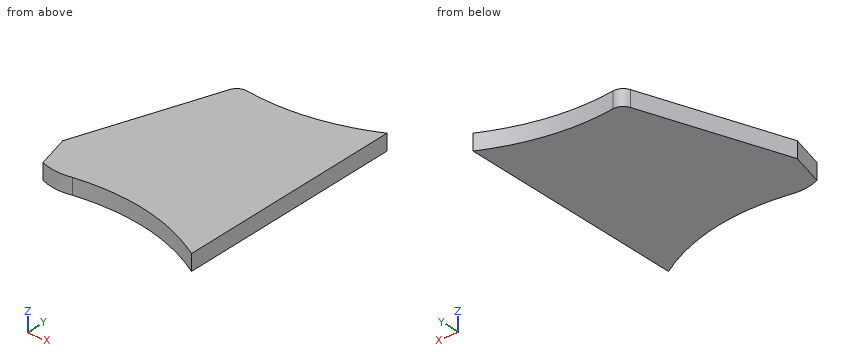
from build123d import *

# Parameters (mm, degrees)
EXTRUDE_1_DEPTH      = 3
EXTRUDE_2_DEPTH      = 3
CUT_EXTRUDE_1_DEPTH  = 10
CUT_EXTRUDE_2_DEPTH  = 10
FILLET_1_R           = 2
CUT_EXTRUDE_3_DEPTH  = 10
CUT_EXTRUDE_4_DEPTH  = 10
CUT_EXTRUDE_5_DEPTH  = 10
CUT_EXTRUDE_6_DEPTH  = 10
CUT_EXTRUDE_7_DEPTH  = 10
EXTRUDE_3_DEPTH      = 3
EXTRUDE_4_DEPTH      = 3
EXTRUDE_5_DEPTH      = 3
CUT_EXTRUDE_8_DEPTH  = 10
CUT_EXTRUDE_9_DEPTH  = 10
CUT_EXTRUDE_10_DEPTH = 10
EXTRUDE_7_DEPTH      = 3
CUT_EXTRUDE_11_DEPTH = 10
CUT_EXTRUDE_12_DEPTH = 10
CUT_EXTRUDE_13_DEPTH = 10
FILLET_2_R           = 2


with BuildPart() as part:
    # 草图1 → 凸台-拉伸1 (new body)
    with BuildSketch(Plane.XY):
        Polygon((18.419709666, -31.180034248), (-18.99770992, -2.648675004), (-11.516544217, 31.616418832), (-4.12729008, 31.616418832), (18.99770992, 31.616418832), (18.99770992, -31.616418832), align=None)
    extrude(amount=EXTRUDE_1_DEPTH)

    # 草图2 → 凸台-拉伸2 (add)
    with BuildSketch(Plane.XY.offset(3)):
        Polygon((18.99770992, 31.616418832), (18.99770992, 39.616418832), (-11.516544217, 31.616418832), align=None)
    extrude(amount=-EXTRUDE_2_DEPTH)

    # 草图3 → 切除-拉伸1 (cut)
    with BuildSketch(Plane.XY.offset(3)):
        with BuildLine():
            Line((-18.99770992, -2.648675004), (18.419709666, -31.180034248))
            Line((18.419709666, -31.180034248), (18.99770992, -31.616418832))
            add(Edge.make_bspline(
                [(-18.99770992, -2.648675004), (-4.909401081, -6.664762391), (12.96021978, -16.653979791), (18.99770992, -31.616418832)],
                knots=[0, 0, 0, 0, 0.839418351, 0.839418351, 0.839418351, 0.839418351], degree=3))
        make_face()
    extrude(amount=-CUT_EXTRUDE_1_DEPTH, mode=Mode.SUBTRACT)

    # 草图4 → 切除-拉伸2 (cut)
    with BuildSketch(Plane.XY.offset(3)):
        with BuildLine():
            Line((18.99770992, 39.616418832), (-11.516544217, 31.616418832))
            add(Edge.make_bspline(
                [(-11.516544217, 31.616418832), (5.451208804, 29.787696143), (18.99770992, 39.616418832)],
                knots=[0, 0, 0, 1, 1, 1], degree=2))
        make_face()
    extrude(amount=-CUT_EXTRUDE_2_DEPTH, mode=Mode.SUBTRACT)

    # 圆角1
    fillet_1_edges = [part.edges().sort_by_distance(p)[0] for p in [
        (-11.516544217, 31.616418832, 1.5),
        (-18.99770992, -2.648675004, 1.5),
    ]]
    fillet(fillet_1_edges, radius=FILLET_1_R)

    # 草图5 → 切除-拉伸3 (cut)
    with BuildSketch(Plane.XY.offset(3)):
        with BuildLine():
            Line((-15.247678714, 14.527147092), (-18.602325656, -0.837743464))
            ThreePointArc((-18.602325656, -0.837743464), (-18.37793511, -2.26862535), (-17.246477615, -3.172825565))
            add(Edge.make_bspline(
                [(-5.349580984, -8.035622202), (-9.34088255, -6.003793842), (-13.405831379, -4.376501244), (-17.246477615, -3.172825565)],
                knots=[0.580679004, 0.580679004, 0.580679004, 0.580679004, 0.804994854, 0.804994854, 0.804994854, 0.804994854], degree=3))
            Line((-5.349580984, -8.035622202), (-15.247678714, 14.527147092))
        make_face()
    extrude(amount=-CUT_EXTRUDE_3_DEPTH, mode=Mode.SUBTRACT)

    # 草图6 → 切除-拉伸4 (cut)
    with BuildSketch(Plane.XY.offset(3)):
        with BuildLine():
            Line((18.99770992, -31.616418832), (18.99770992, -24.041974817))
            add(Edge.make_bspline(
                [(-5.349580984, -8.035622202), (10.712822768, -10.603879461), (18.99770992, -24.041974817)],
                knots=[0, 0, 0, 1, 1, 1], degree=2))
            add(Edge.make_bspline(
                [(18.99770992, -31.616418832), (14.821194408, -21.265949132), (4.982569087, -13.295348934), (-5.349580984, -8.035622202)],
                knots=[0, 0, 0, 0, 0.580679004, 0.580679004, 0.580679004, 0.580679004], degree=3))
        make_face()
    extrude(amount=-CUT_EXTRUDE_4_DEPTH, mode=Mode.SUBTRACT)

    # 草图7 → 切除-拉伸5 (cut)
    with BuildSketch(Plane.XY.offset(3)):
        with BuildLine():
            Line((-7.501131826, -3.13114999), (-5.349580984, -8.035622202))
            add(Edge.make_bspline(
                [(18.99770992, -24.041974817), (10.712822768, -10.603879461), (-5.349580984, -8.035622202)],
                knots=[0, 0, 0, 1, 1, 1], degree=2))
            Line((18.99770992, -24.041974817), (18.99770992, -15.72868914))
            add(Edge.make_bspline(
                [(-7.501131826, -3.13114999), (8.534248318, -3.706395951), (18.99770992, -15.72868914)],
                knots=[0, 0, 0, 1, 1, 1], degree=2))
        make_face()
    extrude(amount=-CUT_EXTRUDE_5_DEPTH, mode=Mode.SUBTRACT)

    # 草图9 → 切除-拉伸6 (cut)
    with BuildSketch(Plane.XY.offset(3)):
        with BuildLine():
            Line((-15.247678714, 14.527147092), (-5.393109321, 31.338029381))
            add(Edge.make_bspline(
                [(-9.792557358, 31.460050353), (-7.562671253, 31.296266706), (-5.393109321, 31.338029381)],
                knots=[0, 0, 0, 1, 1, 1], degree=2))
            ThreePointArc((-9.792557358, 31.460050353), (-11.135472525, 31.068108787), (-11.893031771, 29.892037648))
            Line((-11.893031771, 29.892037648), (-15.247678714, 14.527147092))
        make_face()
    extrude(amount=-CUT_EXTRUDE_6_DEPTH, mode=Mode.SUBTRACT)

    # 草图10 → 切除-拉伸7 (cut)
    with BuildSketch(Plane.XY.offset(3)):
        Polygon((-15.247678714, 14.527147092), (-5.393109321, 31.338029381), (-13.423981873, 10.370019914), align=None)
    extrude(amount=-CUT_EXTRUDE_7_DEPTH, mode=Mode.SUBTRACT)

    # 草图11 → 凸台-拉伸3 (add)
    with BuildSketch(Plane.XY.offset(3)):
        Polygon((-13.423981873, 3.619434962), (-7.501131826, -3.13114999), (-13.423981873, 10.370019914), align=None)
        Polygon((-13.423981873, 16.619434962), (-13.423981873, 10.370019914), (-5.393109321, 31.338029381), align=None)
    extrude(amount=-EXTRUDE_3_DEPTH)

    # 草图12 → 凸台-拉伸4 (add)
    with BuildSketch(Plane.XY.offset(3)):
        with BuildLine():
            Line((18.99770992, -15.72868914), (18.99770992, -16.37868914))
            add(Edge.make_bspline(
                [(-7.501131826, -3.13114999), (8.231572952, -4.86202672), (18.99770992, -16.37868914)],
                knots=[0, 0, 0, 1, 1, 1], degree=2))
            add(Edge.make_bspline(
                [(-7.501131826, -3.13114999), (8.534248318, -3.706395951), (18.99770992, -15.72868914)],
                knots=[0, 0, 0, 1, 1, 1], degree=2))
        make_face()
    extrude(amount=-EXTRUDE_4_DEPTH)

    # 草图14 → 凸台-拉伸5 (add)
    with BuildSketch(Plane.XY.offset(3)):
        Polygon((-13.423981873, 16.619434962), (-5.393109321, 31.338029381), (-15.088083527, 18.619208438), (-15.088083527, 3.619434962), (-7.501131826, -3.13114999), (-13.423981873, 3.619434962), align=None)
    extrude(amount=-EXTRUDE_5_DEPTH)

    # 草图15 → 切除-拉伸8 (cut)
    with BuildSketch(Plane.XY.offset(3)):
        Polygon((-5.393109321, 31.338029381), (-15.088083527, 18.619208438), (-15.088083527, 14.468365238), align=None)
    extrude(amount=-CUT_EXTRUDE_8_DEPTH, mode=Mode.SUBTRACT)

    # 草图16 → 切除-拉伸9 (cut)
    with BuildSketch(Plane.XY.offset(3)):
        with BuildLine():
            Line((18.99770992, -16.37868914), (18.99770992, -10.902642973))
            add(Edge.make_bspline(
                [(-7.501131826, -3.13114999), (7.093543529, -2.593480943), (18.99770992, -10.902642973)],
                knots=[0, 0, 0, 1, 1, 1], degree=2))
            add(Edge.make_bspline(
                [(-7.501131826, -3.13114999), (8.231572952, -4.86202672), (18.99770992, -16.37868914)],
                knots=[0, 0, 0, 1, 1, 1], degree=2))
        make_face()
    extrude(amount=-CUT_EXTRUDE_9_DEPTH, mode=Mode.SUBTRACT)

    # 草图17 → 切除-拉伸10 (cut)
    with BuildSketch(Plane.XY.offset(3)):
        with BuildLine():
            Line((18.99770992, -10.902642973), (18.99770992, -8.085223828))
            add(Edge.make_bspline(
                [(-7.501131826, -3.13114999), (6.687210299, -0.804092069), (18.99770992, -8.085223828)],
                knots=[0, 0, 0, 1, 1, 1], degree=2))
            add(Edge.make_bspline(
                [(18.99770992, -10.902642973), (7.093543529, -2.593480943), (-7.501131826, -3.13114999)],
                knots=[0, 0, 0, 1, 1, 1], degree=2))
        make_face()
    extrude(amount=-CUT_EXTRUDE_10_DEPTH, mode=Mode.SUBTRACT)

    # 草图18 → 凸台-拉伸7 (add)
    with BuildSketch(Plane.XY.offset(3)):
        with BuildLine():
            Line((-15.088083527, 3.619434962), (-13.3809595, -2.744921014))
            add(Edge.make_bspline(
                [(-13.3809595, -2.744921014), (-10.489009144, -3.877027088), (-7.501131826, -3.13114999)],
                knots=[0, 0, 0, 1, 1, 1], degree=2))
            Line((-7.501131826, -3.13114999), (-15.088083527, 3.619434962))
        make_face()
    extrude(amount=-EXTRUDE_7_DEPTH)

    # 草图19 → 切除-拉伸11 (cut)
    with BuildSketch(Plane.XY.offset(3)):
        Polygon((-13.593259145, 17.069422728), (-15.088083527, 14.468365238), (-15.088083527, 11.468365238), align=None)
    extrude(amount=-CUT_EXTRUDE_11_DEPTH, mode=Mode.SUBTRACT)

    # 草图20 → 切除-拉伸12 (cut)
    with BuildSketch(Plane.XY.offset(3)):
        with BuildLine():
            Line((18.99770992, 35.207268429), (18.99770992, 39.616418832))
            add(Edge.make_bspline(
                [(-5.393109321, 31.338029381), (7.941746813, 31.594716807), (18.99770992, 39.616418832)],
                knots=[0, 0, 0, 1, 1, 1], degree=2))
            add(Edge.make_bspline(
                [(-5.393109321, 31.338029381), (7.395374053, 29.358468499), (18.99770992, 35.207268429)],
                knots=[0, 0, 0, 1, 1, 1], degree=2))
        make_face()
    extrude(amount=-CUT_EXTRUDE_12_DEPTH, mode=Mode.SUBTRACT)

    # 草图22 → 切除-拉伸13 (cut)
    with BuildSketch(Plane.XY.offset(3)):
        Polygon((-5.393109324, 31.338029381), (-15.088083527, 3.619434962), (-15.088083527, 11.468365238), (-13.593259145, 17.069422728), align=None)
    extrude(amount=-CUT_EXTRUDE_13_DEPTH, mode=Mode.SUBTRACT)

    # 圆角2
    fillet_2_edges = [part.edges().sort_by_distance(p)[0] for p in [
        (-5.393109321, 31.338029381, 1.5),
    ]]
    fillet(fillet_2_edges, radius=FILLET_2_R)


solid = part.part
Geometry check sheet. Reference: the model listing, model coordinates, mm. Give positions to 0.01 mm unless a question says otherwise; leave off trailing zeros. Loops run counter-clockwise (first coordinate to the right, second up) from the corner with the lowest first, then second, coordinate; pieces in that order, holes last. Notation, with made-up numbers: (-25.5, 70) -> (32.5, 70) arc R17 cw to (32.5, 93) -> close; hole circle Ø4 at (78.5, 16). An arc over 180 degrees is marked (long way). Answer in a Markdown table with one row per item. Add a question column.
1) Cross-section at B-B on y = 8. Record the boundary of the cut face in (x, z), and give its area (3 significant figures).
2) Cross-section at A-A on y = 25. Record the boundary of the cut face in (x, z), and give its area (3 significant figures).
3) Material ranges on probe 1 along Y at (x, z) = (8, 1.45); probe 2 along X at (y, z) = (7.5, 1.65); probe 3 along Y at (x, z) = (15.5, 0.85), recorded low to high. Write a range as from..to.
Outcome:
| question | item | result |
|---|---|---|
| 1 | outline | (-13.56, 0) -> (19, 0) -> (19, 3) -> (-13.56, 3) -> close |
| 1 | area | 97.7 mm^2 |
| 2 | outline | (-7.61, 0) -> (19, 0) -> (19, 3) -> (-7.61, 3) -> close |
| 2 | area | 79.8 mm^2 |
| 3 | probe 1 | y = -3.58..31.47 |
| 3 | probe 2 | x = -13.73..19 |
| 3 | probe 3 | y = -6.23..33.63 |
